from build123d import *

# Parameters (mm, degrees)
EXTRUDE_2_DEPTH = 80
SKETCH_1_R      = 8
EXTRUDE_3_DEPTH = 82.5


with BuildPart() as part:
    # Sketch 3D_1 → 보스-돌출2 (new body)
    with BuildSketch(Plane(origin=(-57.5, 0, 62.5), x_dir=(0.6770565308208834, 0, -0.7359310117618296), z_dir=(0, -1, 0))):
        Polygon((0, 0), (77.861501044, 84.632066353), (169.852877515, 0), (91.99137647, -84.632066353), align=None)
    extrude(amount=-EXTRUDE_2_DEPTH)

    # 스케치1 → 보스-돌출3 (add, symmetric)
    with BuildSketch(Plane(origin=(0, 0, 0), x_dir=(0, 0, -1), z_dir=(1, 0, 0))):
        with Locations((-35, 15)):
            Circle(SKETCH_1_R)
    extrude_3 = extrude(amount=EXTRUDE_3_DEPTH, both=True)

    # 대칭 복사1: 보스-돌출3 across plane
    add(extrude_3.mirror(Plane.XY))


solid = part.part
Verification items for the finished model (mm, model axes). A direction names the side the tool comes from. Give positions to 0.01 mm unless a question says otherwise; leave off trailing zeros. Write each loop counter-clockwise with the first axis right and the second up, starting at its lowest first coordinate (ties: lowest second). Pieces come first, ordered by that corner, then holes.
(1) Cross-section at C-C (z = 35). Enter the section's corners in (x, y).
(2) Access from +Z, -Z, +X, -X, +Y, -Y to the whole of each face (thin tool, end or side, straight path). Record for faces 1 (the face through (70.175, 10.132, -41.349)), 2 (the face through (2, 80, 0)), 3 (the face through (-69.825, 10.132, -41.349)).
(3) Gauge pin test, flat ends, axial feed: pin 1 (8 mm diameter, centred on y = 39.5, z = 32, fed in from -X); pin 2 (1.5 mm diameter, centred on y = 54, z = -41.5, fed in from +X). Record the tip position at first contact, or that the pin passes through.
(4) Cross-section at D-D (y = 45.5). Enter the section's corners in (x, z), plus the area to 3 significant figures.
(5) Cross-section at B-B (x = -61). Enter the section's corners in (y, z).
(6) Material ranges on line 1 (X direction, y = 22, z = 28), recorded low to high.
(7) Cross-section at A-A (y = 15). Enter the section's corners in (x, z), plus the area to 3 significant figures.
Worked out:
1. outline: (-82.5, 7) - (-57.5, 7) - (-57.5, 0) - (57.5, 0) - (57.5, 7) - (82.5, 7) - (82.5, 23) - (57.5, 23) - (57.5, 80) - (-57.5, 80) - (-57.5, 23) - (-82.5, 23) - close
2. face 1: +X
2. face 2: +Z, -Z, +X, -X, +Y
2. face 3: -X
3. pin 1: stops at x = -57.5
3. pin 2: stops at x = 57.5
4. outline: (-57.5, -62.5) - (57.5, -62.5) - (57.5, 62.5) - (-57.5, 62.5) - close
4. area: 14,400 mm2
5. outline: circle Ø16 at (15, -35); circle Ø16 at (15, 35)
6. line 1: x = -57.5 to 57.5
7. outline: (-82.5, -43) - (-57.5, -43) - (-57.5, -62.5) - (57.5, -62.5) - (57.5, -43) - (82.5, -43) - (82.5, -27) - (57.5, -27) - (57.5, 27) - (82.5, 27) - (82.5, 43) - (57.5, 43) - (57.5, 62.5) - (-57.5, 62.5) - (-57.5, 43) - (-82.5, 43) - (-82.5, 27) - (-57.5, 27) - (-57.5, -27) - (-82.5, -27) - close
7. area: 16,000 mm2
